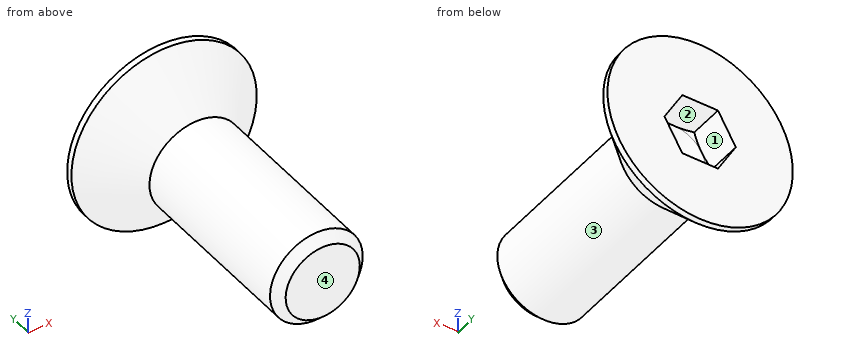
from build123d import *

# Parameters (mm, degrees)
CUT_EXTRUDE2_REACH = 10.791


with BuildPart() as part:
    # Sketch1 → Revolve1 (revolve)
    with BuildSketch(Plane.XY, mode=Mode.PRIVATE) as revolve1_sk:
        Polygon((-1.5, -1.7), (-1.5, -7.4), (-1.2, -7.7), (0, -7.7), (0, -1.7), (-1, -1.2), (-1, 0), (-3, 0), (-3, -0.2), align=None)
    revolve(revolve1_sk.sketch.rotate(Axis((0, 2.75, 0), (0, -1, 0)), 270), axis=Axis((0, 2.75, 0), (0, -1, 0)))

    # Cut-Extrude2: up to this cone (the profile starts inside it)
    cut_extrude2_end = Plane(origin=(0, 0, 0), z_dir=(0, 1, 0)).offset(-1.699999) * Cone(2e-06, 32.782, 16.390999, align=(Align.CENTER, Align.CENTER, Align.MIN), mode=Mode.PRIVATE)
    # Sketch3 → Cut-Extrude2 (cut, up to the surface)
    with BuildSketch(Plane(origin=(0, 0, 0), x_dir=(1, 0, 0), z_dir=(0, 1, 0)), mode=Mode.PRIVATE) as cut_extrude2_sk1:
        Polygon((-0.577350269, -1), (0.577350269, -1), (1.154700538, 0), (0.577350269, 1), (-0.577350269, 1), (-1.154700538, 0), align=None)
    cut_extrude2_tool1 = extrude(cut_extrude2_sk1.sketch, amount=-CUT_EXTRUDE2_REACH, mode=Mode.PRIVATE) & cut_extrude2_end
    add(cut_extrude2_tool1.solids().sort_by_distance((0, 0, 0))[0], mode=Mode.SUBTRACT)


solid = part.part
Geometry check sheet. Reference: the model listing, model coordinates, mm. Face numbers are marked on the shaded views. Give positions to 0.01 mm unless a question says otherwise; leave off trailing zeros. Order: outer loops, then holes, each group sorted by start corner. A loop starts at its lowest first (then second) coordinate and runs counter-clockwise, first axis right, second up.
1. Depth check by flat-ended pin: pin 1 (3 mm diameter, centred on y = -5.5, z = 1.5, fed in from -X); pin 2 (1 mm diameter, centred on y = -5, z = 1, fed in from +X). Enter the tip coordinate at first touch or a pass-through.
Completed:
pin 1: stops at x = -1.5
pin 2: stops at x = 1.41
2. Scan lines: line 1 (X direction, y = -0.5, z = -0.95); line 2 (X direction, y = -5, z = 0.45); line 3 (Y direction, x = 2.75, z = 0.2). Record each from-to range of solid material in increasing order.
Completed:
line 1: x = -2.53 to -0.61, 0.61 to 2.53
line 2: x = -1.43 to 1.43
line 3: y = -0.44 to 0
3. Sectioned sample at B-B (y = -5.25). Record the boundary of the cut face in (x, z).
Completed:
outline: circle Ø3 at (0, 0)
4. Sectioned sample at A-A (y = -1.5). Record the boundary of the cut face in (x, z).
Completed:
outline: circle Ø3.4 at (0, 0); hole circle Ø0.8 at (0, 0)
5. Draft check along X on the marked faces 1, 2, 3 and 4. Enter one of: pulls with the +X half, pulls with the -X half, needs draft (parallel to the pull), parting line crosses it, or undercut.
Completed:
face 1: undercut
face 2: undercut
face 3: parting line crosses it
face 4: needs draft
